The listing builds one solid part. Answer for the finished solid, in the listing's coordinates (mm). Round coordinates to 2 decimals unless told otherwise and drop trailing zeros. Loops run counter-clockwise (first coordinate to the right, second up) from the corner with the lowest first, then second, coordinate; pieces in that order, holes last. Notation, with made-up numbers: (32, 81) -> (90, 81) arc R18 cw to (90, 110) -> close; hole circle Ø7 at (1.5, 0). An arc over 180 degrees is marked (long way). Write each question's results on one line, items separated by ' | '. Start each with the question number.
(1) Straight lines are drawn through the part: probe 1 along Z at (x, y) = (2.75, -12); probe 2 along X at (y, z) = (4.5, -3); probe 3 along X at (y, z) = (8.5, -5.5). For each, find the intervals that lie inside material, in ascending order.
(2) Flat-ended cylindrical pins translate along their axes: pin 1 (5 mm diameter, centred on y = 0, z = 4, fed in from +X); pin 2 (6 mm diameter, centred on x = 3.5, y = -7, fed in from -Z); pin 3 (12 mm diameter, centred on x = -0.5, y = 13, fed in from +Z). Find the tip coordinate at first contact, or state that the pin passes through.
(3) The part is cut by section B-B (y = -6). Determine the outline of the cut face in (x, z).
(4) The part is cut by section A-A (y = 2). Determine the outline of the cut face in (x, z), plus the area to 3 significant figures.
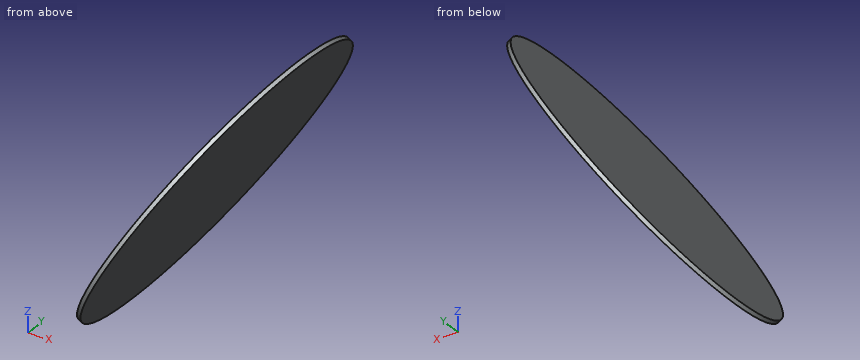
```python
from build123d import *

# Parameters (mm, degrees)
SKETCH1_R             = 40
BOSS_EXTRUDE1_DEPTH   = 1
SCALE1_SCALE          = 0.5
BODY_MOVE_COPY3_ANGLE = 30


with BuildPart() as part:
    # Sketch1 → Boss-Extrude1 (new body)
    with BuildSketch(Plane(origin=(0, 0, 0), x_dir=(0, 0, -1), z_dir=(1, 0, 0))):
        Circle(SKETCH1_R)
    extrude(amount=BOSS_EXTRUDE1_DEPTH)


with BuildPart() as part_1:
    # Scale1: scaled about (0.5, 0, 0)
    add(part.part.scale(SCALE1_SCALE).moved(Location((0.25, 0, 0))))


with BuildPart() as part_2:
    # Body-Move/Copy2: moved
    add(part_1.part.moved(Location((4.171055646, 0, 0))))


with BuildPart() as part_3:
    # Body-Move/Copy3: moved
    add(part_2.part.rotate(Axis((7.238444841, 0, -0.038800486), (0, 1, 0)), BODY_MOVE_COPY3_ANGLE))


solid = part_3.part
```
Checked values:
1) probe 1: z = -3.18 to -2.18 | probe 2: x = 2.28 to 2.85 | probe 3: x = 0.83 to 1.41
2) pin 1: stops at x = 8.34 | pin 2: stops at z = -7.08 | pin 3: stops at z = 2.58
3) outline: (-4.72, -15.12) -> (-4.29, -15.37) -> (14.79, 17.68) -> (14.36, 17.93) -> close
4) outline: (-5.13, -15.83) -> (-4.7, -16.08) -> (15.2, 18.39) -> (14.77, 18.64) -> close | area: 19.9 mm2
